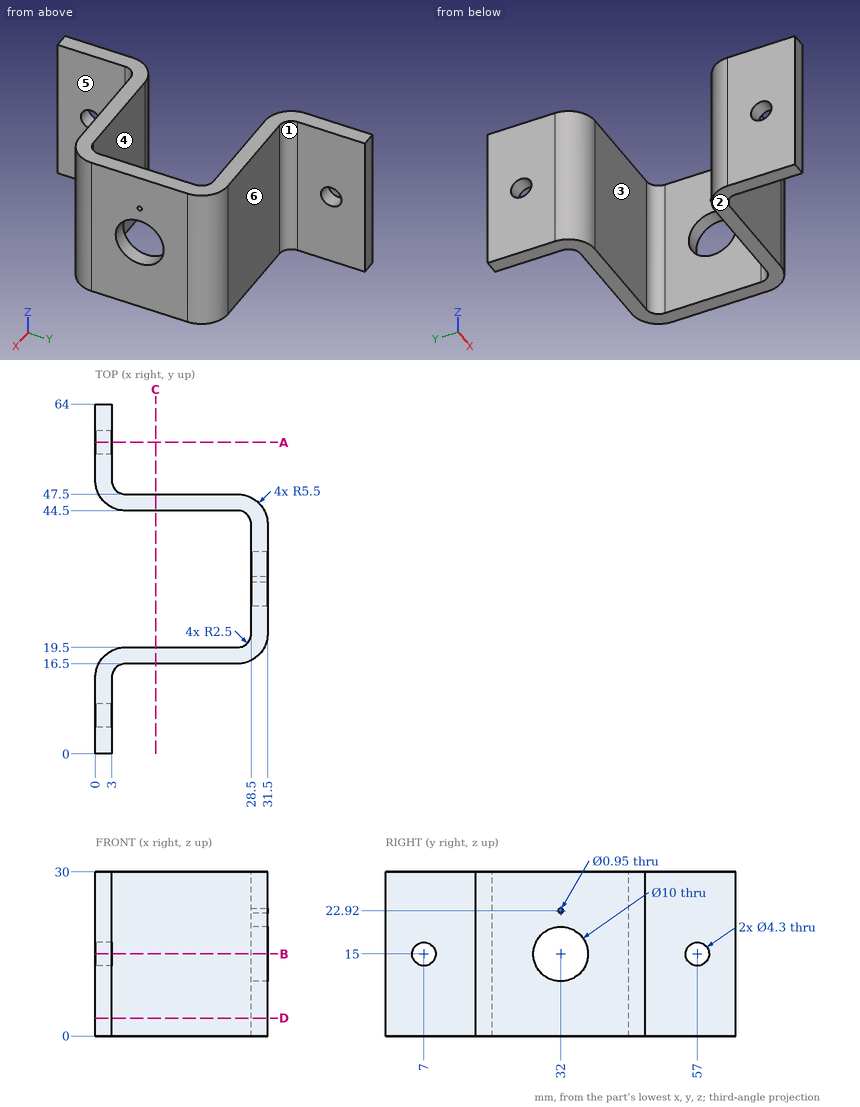
Geometry check sheet. Reference: drawing and pictorial views, mm from the part's lowest x, y, z. A direction names the side the tool comes from. Give positions to 0.01 mm unless a question says otherwise; leave off trailing zeros. Loops run counter-clockwise (first coordinate to the right, second up) from the corner with the lowest first, then second, coordinate; pieces in that order, holes last. Notation, with made-up numbers: (57.25, -18.5) - (88.25, -18.5) arc R20 cw to (88.25, -7.5) - close; hole circle Ø2 at (72, 45). An arc over 180 degrees is marked (long way). One line per question, with ' | ' between items. Start each with the question number.
1. Material ranges on line 1 along Y through (x, z) = (9, 19); line 2 along Y through (x, z) = (1, 15); line 3 along Y through (x, z) = (1.95, 15), recorded low to high. Write a range as [from, to].
2. Cross-section at D-D, the plane z = 3.25. Enter the section's corners in (x, y), plus the area to 3 significant figures.
3. Set-up check for the marked faces 4, 5 and 6: record each of +Z, -Z, +X, -X, +Y, -Y from which the full face is reachable in a straight line by a thin tool's end or side.
4. Gauge pin test, flat ends, axial feed: pin 1 Ø1.5 at (x, z) = (11.5, 6.5) entering from +Y; pin 2 Ø7 at (y, z) = (57, 20.5) entering from +X; pin 3 Ø10 at (y, z) = (31, 19.5) entering from -X; pin 4 Ø4 at (y, z) = (7, 15) entering from -X. Record the tip position at first contact, or that the pin passes through.
5. Cross-section at A-A, the plane y = 57. Enter the section's corners in (x, z), plus the area to 3 significant figures.
6. Draft check along Y on the marked faces 1, 2 and 3. Enter one of: released by +Y, released by -Y, zero draft, split by the parting line, or undercut.
7. Cross-section at B-B, the plane z = 15. Give the number of separate pieces and of enclosed holes in the cut face, plus the area to 3 significant figures.
8. Cross-section at C-C, the plane x = 11. Enter the section's corners in (y, z), plus the area to 3 significant figures.
Check result:
1) line 1: y = [16.5, 19.5], [44.5, 47.5] | line 2: y = [0, 4.85], [9.15, 17.16], [46.84, 54.85], [59.15, 64] | line 3: y = [0, 4.85], [9.15, 18.2], [45.8, 54.85], [59.15, 64]
2) outline: (0, 0) - (3, 0) - (3, 14) arc R2.5 cw to (5.5, 16.5) - (26, 16.5) arc R5.5 ccw to (31.5, 22) - (31.5, 42) arc R5.5 ccw to (26, 47.5) - (5.5, 47.5) arc R2.5 cw to (3, 50) - (3, 64) - (0, 64) - (0, 50) arc R5.5 ccw to (5.5, 44.5) - (26, 44.5) arc R2.5 cw to (28.5, 42) - (28.5, 22) arc R2.5 cw to (26, 19.5) - (5.5, 19.5) arc R5.5 ccw to (0, 14) - close | area: 342 mm2
3) face 4: +Z, -Z, -X | face 5: +Z, -Z, +X, -Y | face 6: +Z, -Z, +X, +Y
4) pin 1: stops at y = 47.5 | pin 2: stops at x = 3 | pin 3: stops at x = 28.5 | pin 4: passes through
5) outline: (0, 0) - (3, 0) - (3, 12.85) - (0, 12.85) - close; (0, 17.15) - (3, 17.15) - (3, 30) - (0, 30) - close | area: 77.1 mm2
6) face 1: released by +Y | face 2: zero draft | face 3: undercut
7) separate pieces: 4 | enclosed holes: 0 | area: 287 mm2
8) outline: (16.5, 0) - (19.5, 0) - (19.5, 30) - (16.5, 30) - close; (44.5, 0) - (47.5, 0) - (47.5, 30) - (44.5, 30) - close | area: 180 mm2
